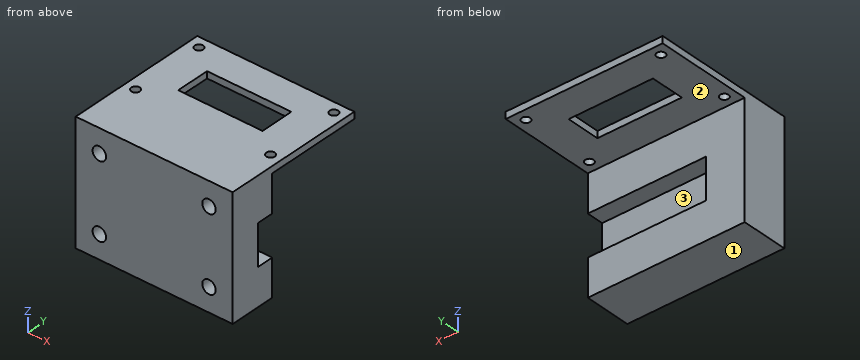
from build123d import *

# Parameters (mm, degrees)
SKETCH1_W           = 46.5
SKETCH1_H           = 34
BOSS_EXTRUDE1_DEPTH = 13.75
SKETCH2_W           = 46.5
SKETCH2_H           = 42.25
BOSS_EXTRUDE2_DEPTH = 2
CUT_EXTRUDE1_REACH  = 62.18
SKETCH3_R           = 1.25
SKETCH3_W           = 25
SKETCH3_H           = 10
SKETCH4_W           = 35
SKETCH4_H           = 12
CUT_EXTRUDE2_DEPTH  = 5
SKETCH6_R           = 2
CUT_EXTRUDE3_DEPTH  = 10


with BuildPart() as part:
    # Sketch1 → Boss-Extrude1 (new body)
    with BuildSketch(Plane(origin=(0, 0, 0), x_dir=(1, 0, 0), z_dir=(0, 1, 0))):
        Rectangle(SKETCH1_W, SKETCH1_H)
    extrude(amount=BOSS_EXTRUDE1_DEPTH)

    # Sketch2 → Boss-Extrude2 (add)
    with BuildSketch(Plane.XY.offset(17)):
        with Locations((0, 21.125)):
            Rectangle(SKETCH2_W, SKETCH2_H)
    extrude(amount=BOSS_EXTRUDE2_DEPTH)

    # Sketch3 → Cut-Extrude1 (cut, up to next)
    with BuildSketch(Plane.XY.offset(19), mode=Mode.PRIVATE) as cut_extrude1_sk1:
        with Locations((-20, 39)):
            Circle(SKETCH3_R)
    cut_extrude1_tool1 = extrude(cut_extrude1_sk1.sketch, amount=-CUT_EXTRUDE1_REACH, mode=Mode.PRIVATE) & part.part
    # Sketch3 → Cut-Extrude1 (cut, up to next)
    with BuildSketch(Plane.XY.offset(19), mode=Mode.PRIVATE) as cut_extrude1_sk2:
        with Locations(Location((20, 39, 0), (0, 0, 180))):
            Circle(SKETCH3_R)
    cut_extrude1_tool2 = extrude(cut_extrude1_sk2.sketch, amount=-CUT_EXTRUDE1_REACH, mode=Mode.PRIVATE) & part.part
    # Sketch3 → Cut-Extrude1 (cut, up to next)
    with BuildSketch(Plane.XY.offset(19), mode=Mode.PRIVATE) as cut_extrude1_sk3:
        with Locations((20, 17)):
            Circle(SKETCH3_R)
    cut_extrude1_tool3 = extrude(cut_extrude1_sk3.sketch, amount=-CUT_EXTRUDE1_REACH, mode=Mode.PRIVATE) & part.part
    # Sketch3 → Cut-Extrude1 (cut, up to next)
    with BuildSketch(Plane.XY.offset(19), mode=Mode.PRIVATE) as cut_extrude1_sk4:
        with Locations(Location((-20, 17, 0), (0, 0, 180))):
            Circle(SKETCH3_R)
    cut_extrude1_tool4 = extrude(cut_extrude1_sk4.sketch, amount=-CUT_EXTRUDE1_REACH, mode=Mode.PRIVATE) & part.part
    # Sketch3 → Cut-Extrude1 (cut, up to next)
    with BuildSketch(Plane.XY.offset(19), mode=Mode.PRIVATE) as cut_extrude1_sk5:
        with Locations((0, 28)):
            Rectangle(SKETCH3_W, SKETCH3_H)
    cut_extrude1_tool5 = extrude(cut_extrude1_sk5.sketch, amount=-CUT_EXTRUDE1_REACH, mode=Mode.PRIVATE) & part.part
    add(cut_extrude1_tool1.solids().sort_by_distance((-20, 39, 19))[0], mode=Mode.SUBTRACT)
    add(cut_extrude1_tool2.solids().sort_by_distance((20, 39, 19))[0], mode=Mode.SUBTRACT)
    add(cut_extrude1_tool3.solids().sort_by_distance((20, 17, 19))[0], mode=Mode.SUBTRACT)
    add(cut_extrude1_tool4.solids().sort_by_distance((-20, 17, 19))[0], mode=Mode.SUBTRACT)
    add(cut_extrude1_tool5.solids().sort_by_distance((0, 28, 19))[0], mode=Mode.SUBTRACT)

    # Sketch4 → Cut-Extrude2 (cut)
    with BuildSketch(Plane(origin=(0, 13.75, 0), x_dir=(1, 0, 0), z_dir=(0, 1, 0))):
        with Locations((5.75, 0)):
            Rectangle(SKETCH4_W, SKETCH4_H)
    extrude(amount=-CUT_EXTRUDE2_DEPTH, mode=Mode.SUBTRACT)

    # Sketch6 → Cut-Extrude3 (cut)
    with BuildSketch(Plane.XZ):
        with Locations(Location((16.25, -10, 0), (0, 0, 270))):
            Circle(SKETCH6_R)
        with Locations(Location((16.25, 12, 0), (0, 0, 270))):
            Circle(SKETCH6_R)
        with Locations(Location((-16.25, -10, 0), (0, 0, 270))):
            Circle(SKETCH6_R)
        with Locations(Location((-16.25, 12, 0), (0, 0, 270))):
            Circle(SKETCH6_R)
    extrude(amount=-CUT_EXTRUDE3_DEPTH, mode=Mode.SUBTRACT)


solid = part.part
Verification items for the finished model (mm, model axes). Face numbers are marked on the shaded views. A direction names the side the tool comes from. Coordinates: 2 decimals unless noted, no trailing zeros. Loops run counter-clockwise (first coordinate to the right, second up) from the corner with the lowest first, then second, coordinate; pieces in that order, holes last. Notation, with made-up numbers: (24, -21.75) -> (64, -21.75) arc R13 ccw to (64, -5.75) -> close; hole circle Ø9 at (-34, 15.5). An arc over 180 degrees is marked (long way). Answer as a JSON object with one key per item and string values. Group by question number.
Item 1: Sectioned sample at C-C on x = 7.5. Record the boundary of the cut face in (y, z), plus the area to 3 significant figures.
Item 2: Depth check by flat-ended pin: pin 1 (3 mm diameter, centred on x = -16, z = -10.5, fed in from -Y); pin 2 (3 mm diameter, centred on x = 16, z = 12, fed in from -Y); pin 3 (8 mm diameter, centred on x = -3, z = 11.5, fed in from +Y); pin 4 (14 mm diameter, centred on x = 1, y = 30.5, fed in from -Z). Enter the tip coordinate at first touch or a pass-through.
Item 3: Sectioned sample at D-D on y = 39. Record the boundary of the cut face in (x, z).
Item 4: Scan lines: probe 1 along X at (y, z) = (6.75, 12); probe 2 along Y at (x, z) = (20, 18.3); probe 3 along Y at (x, z) = (-18, -10). Record each from-to range of solid material in increasing order.
Item 5: Sectioned sample at A-A on x = 20. Record the boundary of the cut face in (y, z), plus the area to 3 significant figures.
Item 6: Sectioned sample at B-B on y = 29.5. Record the boundary of the cut face in (x, z), plus the area to 3 significant figures.
Item 7: Tool access check on the marked faces 1, 2 and 3. Record the directions out of +Z, -Z, +X, -X, +Y, -Y that give a thin tool (end or side, any length) a straight path to the whole face; none if there is none.
Evaluation:
{
 "1": {"outline": "(0, -17) -> (13.75, -17) -> (13.75, -6) -> (8.75, -6) -> (8.75, 6) -> (13.75, 6) -> (13.75, 17) -> (23, 17) -> (23, 19) -> (0, 19) -> close; (33, 17) -> (42.25, 17) -> (42.25, 19) -> (33, 19) -> close", "area": "472 mm²"},
 "2": {"pin 1": "stops at y = 0", "pin 2": "stops at y = 10", "pin 3": "stops at y = 13.75", "pin 4": "stops at z = 17"},
 "3": {"outline": "(-23.25, 17) -> (-21.25, 17) -> (-21.25, 19) -> (-23.25, 19) -> close; (-18.75, 17) -> (18.75, 17) -> (18.75, 19) -> (-18.75, 19) -> close; (21.25, 17) -> (23.25, 17) -> (23.25, 19) -> (21.25, 19) -> close"},
 "4": {"probe 1": "x = -23.25 to -18.25, -14.25 to 14.25, 18.25 to 23.25", "probe 2": "y = 0 to 15.75, 18.25 to 37.75, 40.25 to 42.25", "probe 3": "y = 10 to 13.75"},
 "5": {"outline": "(0, -17) -> (13.75, -17) -> (13.75, -6) -> (8.75, -6) -> (8.75, 6) -> (13.75, 6) -> (13.75, 17) -> (15.75, 17) -> (15.75, 19) -> (0, 19) -> close; (18.25, 17) -> (37.75, 17) -> (37.75, 19) -> (18.25, 19) -> close; (40.25, 17) -> (42.25, 17) -> (42.25, 19) -> (40.25, 19) -> close", "area": "482 mm²"},
 "6": {"outline": "(-23.25, 17) -> (-12.5, 17) -> (-12.5, 19) -> (-23.25, 19) -> close; (12.5, 17) -> (23.25, 17) -> (23.25, 19) -> (12.5, 19) -> close", "area": "43.0 mm²"},
 "7": {"face 1": "-Z, +X, -X, +Y, -Y", "face 2": "-Z, +X, -X, +Y", "face 3": "+X, +Y"}
}
